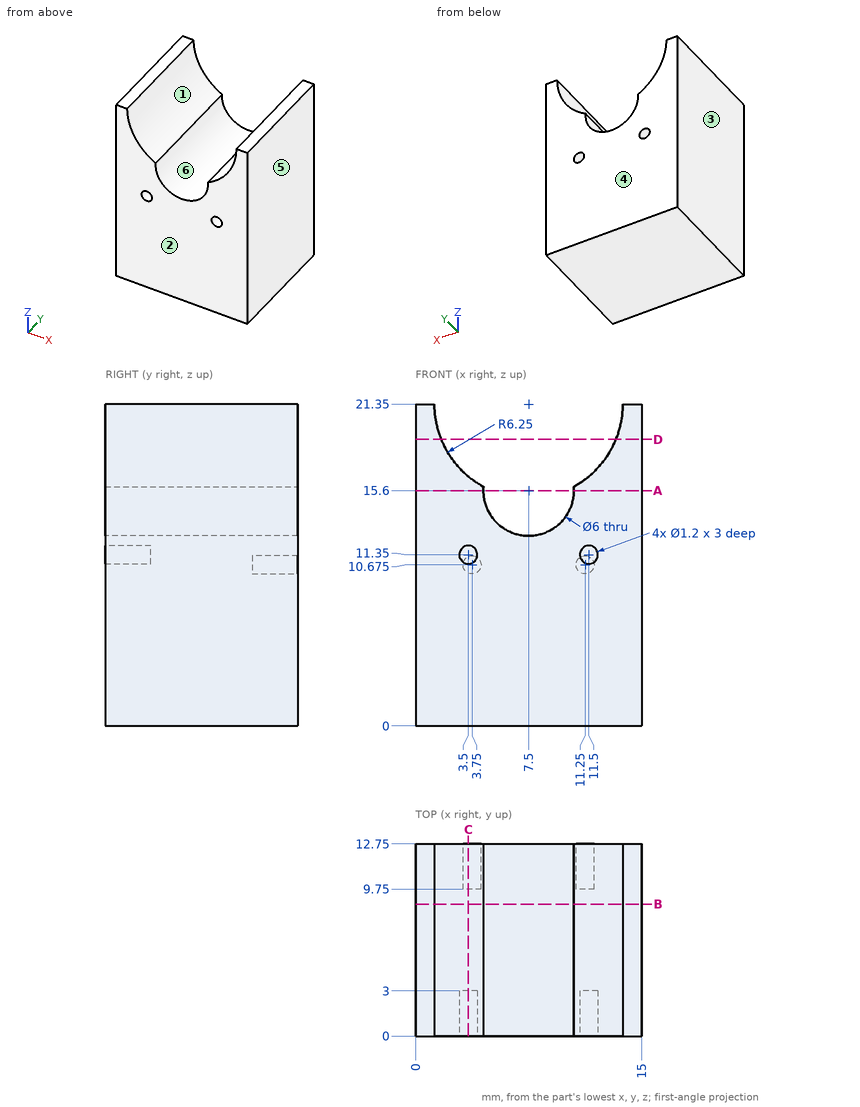
Here's the drawing with two shaded views (mm, measured from the low corner). I have some questions. A direction names the side the tool comes from. Coordinates: 2 decimals unless noted, no trailing zeros. Write each loop counter-clockwise with the first axis right and the second up, starting at its lowest first coordinate (ties: lowest second). Pieces come first, ordered by that corner, then holes. Notation, with made-up numbers: (18, 37.5) -> (39, 37.5) arc R10 ccw to (39, 41.5) -> close; hole circle Ø7 at (3.25, -17). An arc over 180 degrees is marked (long way). Answer as CSV lines item,"result".
1) If we section it at D-D on z = 19: Please give me the cut outline in (x, y), then the cut area to 3 significant figures.
Check result:
outline,"(0, 0) -> (1.71, 0) -> (1.71, 12.75) -> (0, 12.75) -> close; (13.29, 0) -> (15, 0) -> (15, 12.75) -> (13.29, 12.75) -> close"
area,"43.6 mm²"
2) If I drill on line 1 (X direction, y = 1.7, z = 11.35); line 2 (Z direction, x = 6.5, y = 6.5); line 3 (Z direction, x = 12.25, y = 4.25), over which ranges is the centre line in solid material (lowest first)? Write a range as from..to.
Check result:
line 1,"0..2.9, 4.1..10.9, 12.1..15"
line 2,"0..12.77"
line 3,"0..17.29"
3) Will these pins go through, and if not, where does the flat tip stop? P1, Ø1.1, axis at x = 3.5, z = 11.35, coming from the -Y side; P2, Ø2, axis at x = 8.5, y = 6.5, coming from the +Z side.
Check result:
P1,"y = 3"
P2,"z = 13.36"
4) If we section it at B-B on y = 8.75: Please give me the cut outline in (x, z).
Check result:
outline,"(0, 0) -> (15, 0) -> (15, 21.35) -> (13.75, 21.35) arc R6.25 cw to (10.49, 15.86) arc R3 cw (long way) to (4.51, 15.86) arc R6.25 cw to (1.25, 21.35) -> (0, 21.35) -> close"
5) If we mould it in two halves opening along X, with no side actions, what happens to the marked faces 3, 4, 5 and 6? For each: +X half, -X half, draft (parallel to the pull), parting line (faces both ways), or undercut.
Check result:
face 3,"-X half"
face 4,"draft"
face 5,"+X half"
face 6,"undercut"
6) On a 3-axis mill with a long thin cutter (end or side, diameter ignored), from which of +Z, -Z, +X, -X, +Y, -Y can I reach the whole of each face in a straight line? I mean the marked faces 1 and 2. Say none if no direction works.
Check result:
face 1,"+Z, +Y, -Y"
face 2,"+Z, -Z, +X, -X, -Y"
7) If we section it at C-C on x = 3.5: Please give me the cut outline in (y, z).
Check result:
outline,"(0, 0) -> (12.75, 0) -> (12.75, 10.13) -> (9.75, 10.13) -> (9.75, 11.22) -> (12.75, 11.22) -> (12.75, 16.55) -> (0, 16.55) -> (0, 11.95) -> (3, 11.95) -> (3, 10.75) -> (0, 10.75) -> close"
8) If we section it at A-A on z = 15.6: Please give me the cut outline in (x, y), then the cut area to 3 significant figures.
Check result:
outline,"(0, 0) -> (4.5, 0) -> (4.5, 12.75) -> (0, 12.75) -> close; (10.5, 0) -> (15, 0) -> (15, 12.75) -> (10.5, 12.75) -> close"
area,"115 mm²"
